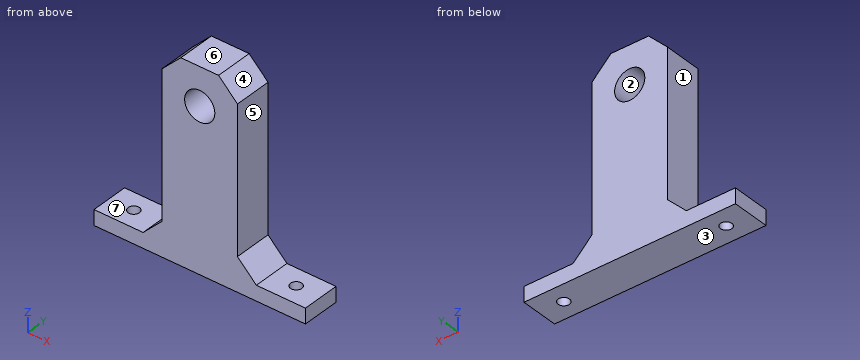
Autodesk Inventor part; units mm, degrees
ref_plane "YZ Plane" through (0, 0, 0) normal (1, 0, 0) x (0, 1, 0)
ref_plane "XZ Plane" through (0, 0, 0) normal (0, 1, 0) x (-1, 0, 0)
ref_plane "XY Plane" through (0, 0, 0) normal (0, 0, 1) x (1, 0, 0)
sketch "Esboço1" plane through (0, 0, 0) normal (0, 0, 1) x (1, 0, 0)
  line L0 (0, 0) -> (56, 0)
  line L1 (56, 0) -> (56, 10)
  line L2 (56, 10) -> (0, 10)
  line L3 (0, 10) -> (0, 0)
  line L4 (18, 10) -> (38, 10)
  line L5 (38, 10) -> (38, 0)
  line L6 (38, 0) -> (18, 0)
  line L7 (18, 0) -> (18, 10)
  line L8 (18, 10) -> (38, 0) construction
  line L9 (38, 10) -> (18, 0) construction
  point P0 (28, 5)
  dimension "d0" = 56
  dimension "d1" = 10
  dimension "d2" = 20
extrude "Extrusão1" add sketch "Esboço1" along normal blind 4 contours L3 L2 L7 L0 | L5 L2 L1 L0
extrude "Extrusão2" add sketch "Esboço1" along normal blind 52.426 contours L7 L2 L5 L0
chamfer "Chanfro1" distance 5 angle 45 4 edges at (38, 5, 4) (18, 5, 4) (38, 5, 52.426) (18, 5, 52.426)
sketch "Esboço2" plane through (0, 10, 0) normal (0, 1, 0) x (1, 0, 0)
  line L0 (33, -52.426) -> (23, -52.426)
  point P0 (0, 0)
  point P1 (28, -42.426)
  dimension "d24" = 10
hole "Furo1" at (28, 10, 42.426) direction (0, -1, 0) diameter 8 end through all
sketch "Esboço3" plane through (0, 0, 4) normal (0, 0, 1) x (1, 0, 0)
  point P0 (0, 0)
  point P1 (6.5, 5)
  point P2 (49.5, 5)
hole "Furo2" at (6.5, 5, 4) at (49.5, 5, 4) direction (0, 0, -1) diameter 3 end through all
properties part number "suporte barra_3DPrint"
Source: CAD feature listing. Evaluate the final solid. Frame: model axes, mm. Face numbers are marked on the shaded views. A direction names the side the tool comes from. Coordinates: 2 decimals unless noted, no trailing zeros. Loops run counter-clockwise (first coordinate to the right, second up) from the corner with the lowest first, then second, coordinate; pieces in that order, holes last. Notation, with made-up numbers: M 85,61.25 L 132,61.25 A20 ccw 132,82.25 Z; hole C 28.5,34 d11. An arc over 180 degrees is marked long. Use CSV: the item, a comma, the result in double quotes.
(1) Contact query for flat-ended pins moving along their axis: pin 1 (4 mm diameter, centred on y = 3, z = 15.5, fed in from -X); pin 2 (2.5 mm diameter, centred on x = 49.5, y = 5, fed in from -Z); pin 3 (5 mm diameter, centred on x = 4, y = 7, fed in from +Z); pin 4 (4 mm diameter, centred on y = 6.5, z = 39.5, fed in from +X). Output: stop coordinate, or through.
Answers follow:
pin 1,"x = 18"
pin 2,"through"
pin 3,"z = 4"
pin 4,"x = 38"
(2) Draft query along X for the marked faces 1, 2, 3 and 4. Return one class per face: pulls with the +X half, pulls with the -X half, needs draft (parallel to the pull), parting line crosses it, or undercut.
Answers follow:
face 1,"pulls with the -X half"
face 2,"undercut"
face 3,"needs draft"
face 4,"pulls with the +X half"
(3) Cut plane D-D on y = 7.75. Return loops of the section in (x, z).
Answers follow:
outline,"M 0,0 L 56,0 L 56,4 L 43,4 L 38,9 L 38,47.43 L 33,52.43 L 23,52.43 L 18,47.43 L 18,9 L 13,4 L 0,4 Z; hole C 28,42.43 d8"
(4) Cut plane A-A on y = 5. Return loops of the section in (x, z), and give its area (3 significant figures).
Answers follow:
outline,"M 0,0 L 5,0 L 5,4 L 0,4 Z; M 8,0 L 48,0 L 48,4 L 43,4 L 38,9 L 38,47.43 L 33,52.43 L 23,52.43 L 18,47.43 L 18,9 L 13,4 L 8,4 Z; M 51,0 L 56,0 L 56,4 L 51,4 Z; hole C 28,42.43 d8"
area,"1,120 mm²"
(5) Line query: line 1 (Y direction, x = 49.5, z = 2.25); line 2 (X direction, y = 5, z = 2.5); line 3 (Z direction, x = 28, y = 7.5). Output: solid intervals per line, ascending. Write a range as [from, to].
Answers follow:
line 1,"[0, 3.5], [6.5, 10]"
line 2,"[0, 5], [8, 48], [51, 56]"
line 3,"[0, 38.43], [46.43, 52.43]"
(6) Cut plane B-B on x = 6.5. Return loops of the section in (y, z), and give its area (3 significant figures).
Answers follow:
outline,"M 0,0 L 3.5,0 L 3.5,4 L 0,4 Z; M 6.5,0 L 10,0 L 10,4 L 6.5,4 Z"
area,"28.0 mm²"
(7) Reachability of the marked faces 5, 6 and 7 from +Z, -Z, +X, -X, +Y, -Y: full face, straight path, thin tool, end or side. Return the list, or none.
Answers follow:
face 5,"+Z, +X, +Y, -Y"
face 6,"+Z, +X, -X, +Y, -Y"
face 7,"+Z, -X, +Y, -Y"
(8) Cut plane C-C on z = 40. Return loops of the section in (x, y).
Answers follow:
outline,"M 18,0 L 24.82,0 L 24.82,10 L 18,10 Z; M 31.18,0 L 38,0 L 38,10 L 31.18,10 Z"
